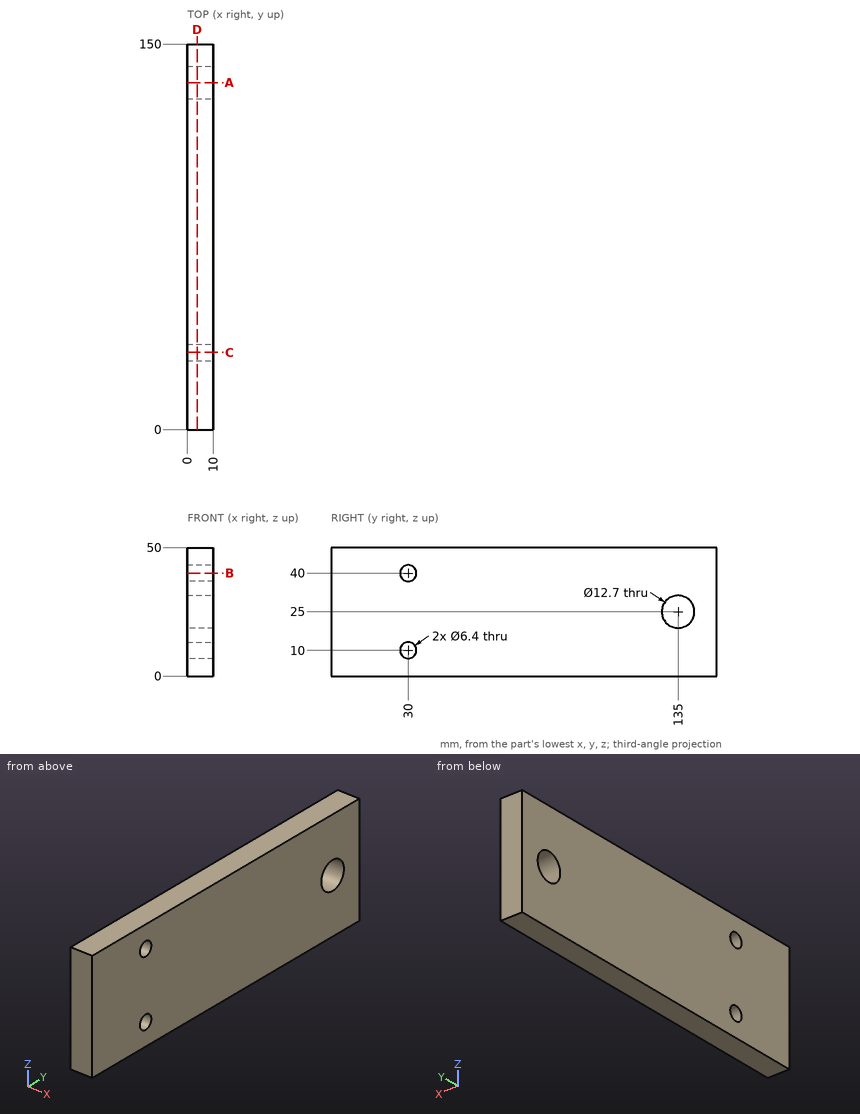
Study the drawing (mm; zero at the part's minimum x, y, z) and answer. Give positions to 0.01 mm unless a question says otherwise; leave off trailing zeros. Write each loop counter-clockwise with the first axis right and the second up, starting at its lowest first coordinate (ties: lowest second). Pieces come first, ordered by that corner, then holes. Notation, with made-up numbers: (45, -0.75) -> (71, -0.75) arc R22 cw to (71, 18.25) -> close; hole circle Ø2 at (21, 4.5). An arc over 180 degrees is marked (long way). Write item = value, one per line.
Q1. A flat-ended cylindrical pin translates along its axis: pin 1 Ø5 at (y, z) = (30, 10) entering from -X. Find the tip coordinate at first contact, or state that the pin passes through.
Computed values:
pin_1 = through
Q2. Section B-B on z = 40 is taken. Determine the outline of the cut face in (x, y), and give its area (3 significant figures).
Computed values:
outline = (0, 0) -> (10, 0) -> (10, 26.8) -> (0, 26.8) -> close; (0, 33.2) -> (10, 33.2) -> (10, 150) -> (0, 150) -> close
area = 1,440 mm^2
Q3. Section D-D on x = 3.75 is taken. Determine the outline of the cut face in (y, z), and give its area (3 significant figures).
Computed values:
outline = (0, 0) -> (150, 0) -> (150, 50) -> (0, 50) -> close; hole circle Ø6.4 at (30, 10); hole circle Ø6.4 at (30, 40); hole circle Ø12.7 at (135, 25)
area = 7,310 mm^2
Q4. Section A-A on y = 135 is taken. Determine the outline of the cut face in (x, z), and give its area (3 significant figures).
Computed values:
outline = (0, 0) -> (10, 0) -> (10, 18.65) -> (0, 18.65) -> close; (0, 31.35) -> (10, 31.35) -> (10, 50) -> (0, 50) -> close
area = 373 mm^2
Q5. Section C-C on y = 30 is taken. Determine the outline of the cut face in (x, z).
Computed values:
outline = (0, 0) -> (10, 0) -> (10, 6.8) -> (0, 6.8) -> close; (0, 13.2) -> (10, 13.2) -> (10, 36.8) -> (0, 36.8) -> close; (0, 43.2) -> (10, 43.2) -> (10, 50) -> (0, 50) -> close
Q6. Consider line 1 along Z through (x, y) = (2.75, 31.5); line 2 along Y through (x, z) = (3, 27); line 3 along Z through (x, y) = (8.25, 137). Determine where each line is inside the solid, lowest interval first.
Computed values:
line_1 = 0 to 7.17, 12.83 to 37.17, 42.83 to 50
line_2 = 0 to 128.97, 141.03 to 150
line_3 = 0 to 18.97, 31.03 to 50
